from build123d import *

# Parameters (mm, degrees)
CROQUIS1_W              = 97
CROQUIS1_H              = 58
SALIENTE_EXTRUIR1_DEPTH = 2
CROQUIS2_W              = 6
CROQUIS2_H              = 6
SALIENTE_EXTRUIR2_DEPTH = 4.2
CROQUIS3_R              = 1.7
CORTAR_EXTRUIR1_DEPTH   = 102.329363957


with BuildPart() as part:
    # Croquis1 → Saliente-Extruir1 (new body)
    with BuildSketch(Plane.XY):
        Rectangle(CROQUIS1_W, CROQUIS1_H)
    extrude(amount=-SALIENTE_EXTRUIR1_DEPTH)

    # Croquis2 → Saliente-Extruir2 (add)
    with BuildSketch(Plane.XY):
        with Locations((-45.5, 26)):
            Rectangle(CROQUIS2_W, CROQUIS2_H)
        with Locations((-45.5, -26)):
            Rectangle(CROQUIS2_W, CROQUIS2_H)
        with Locations((45.5, -26)):
            Rectangle(CROQUIS2_W, CROQUIS2_H)
        with Locations((45.5, 26)):
            Rectangle(CROQUIS2_W, CROQUIS2_H)
    extrude(amount=SALIENTE_EXTRUIR2_DEPTH)

    # Croquis3 → Cortar-Extruir1 (cut, through all)
    with BuildSketch(Plane.ZY.offset(48.5)):
        with Locations(Location((2.011535927, 26.225, 0), (0, 0, 270))):
            Circle(CROQUIS3_R)
        with Locations(Location((2.011535927, -26.225, 0), (0, 0, 270))):
            Circle(CROQUIS3_R)
    extrude(amount=-CORTAR_EXTRUIR1_DEPTH, mode=Mode.SUBTRACT)


solid = part.part
Input: part model. Units: mm. Frame: model coordinates. A direction names the side the tool comes from. Round coordinates to 2 decimals unless told otherwise and drop trailing zeros. Write each loop counter-clockwise with the first axis right and the second up, starting at its lowest first coordinate (ties: lowest second). Pieces come first, ordered by that corner, then holes.
1) Contact query for flat-ended pins moving along their axis: P1, Ø3, axis at y = -19, z = 2, coming from the -X side; P2, Ø12, axis at x = 12.5, y = 20, coming from the +Z side. Output: stop coordinate, or through.
2) Ray query, L1, parallel to Z at x = -19, y = -12; L2, parallel to Y at x = -43.5, z = 0.25. Return the intervals inside material, ascending.
3) Draft query along Z for faces 1 (the flat face through (-11.5, -29, -0.2)), 2 (the flat face through (-1, 0, -2)), 3 (the cylindrical face through (-45.542, 24.655, 1.36)), 4 (the flat face through (45, 26, 4.2)). Return one class per face: pulls with the +Z half, pulls with the -Z half, needs draft (parallel to the pull), parting line crosses it, or undercut.
4) Reachability of faces 5 (the flat face through (-48.5, -0.4, -0.3)), 6 (the flat face through (45, 23, 2)), 7 (the flat face through (42.5, -26, 4)) from +Z, -Z, +X, -X, +Y, -Y: full face, straight path, thin tool, end or side. Return the list, or none.
5) Cut plane A-A (x = -21). Return the cut outline in (y, z), then the cut area to 3 significant figures.
6) Cut plane B-B (y = 20). Return the cut outline in (x, z).
Geometry says:
1. P1: passes through
1. P2: stops at z = 0
2. L1: z = -2 to 0
2. L2: y = -29 to -23, 23 to 29
3. face 1: needs draft
3. face 2: pulls with the -Z half
3. face 3: undercut
3. face 4: pulls with the +Z half
4. face 5: +Z, -Z, -X, +Y, -Y
4. face 6: +Z, +X, -X
4. face 7: +Z, +Y, -Y
5. outline: (-29, -2) - (29, -2) - (29, 0) - (-29, 0) - close
5. area: 116 mm2
6. outline: (-48.5, -2) - (48.5, -2) - (48.5, 0) - (-48.5, 0) - close
